Input: part model. Units: mm. Frame: model coordinates. A direction names the side the tool comes from. Coordinates: 2 decimals unless noted, no trailing zeros. Loops run counter-clockwise (first coordinate to the right, second up) from the corner with the lowest first, then second, coordinate; pieces in that order, holes last. Notation, with made-up numbers: (-35.5, 72.5) - (-8.5, 72.5) arc R13 ccw to (-8.5, 81.5) - close; hole circle Ø11 at (23, 53). An arc over 180 degrees is marked (long way). Write item = value, one per line. Start each with the question number.
from build123d import *

# Parameters (mm, degrees)
CHAMFER1_SIZE = 0.5


with BuildPart() as part:
    # Sketch1 → Revolve1 (revolve)
    with BuildSketch(Plane.XY):
        Polygon((3.925, 17.592522397), (6.15, 17.592522397), (6.15, 13.092522397), (9.15, 13.092522397), (9.15, 18.092522397), (11.15, 18.092522397), (11.15, 11.092522397), (9.662817283, 11.092522397), (3.925, 11.092522397), align=None)
    revolve(axis=Axis((0, 0, 0), (0, 1, 0)))

    # Chamfer1
    chamfer1_edges = [part.edges().sort_by_distance(p)[0] for p in [
        (-11.15, 18.092522397, 0),
        (-11.15, 11.092522397, 0),
    ]]
    chamfer(chamfer1_edges, length=CHAMFER1_SIZE)


solid = part.part
Item 1: Cut plane B-B on z = 0. Return loops of the section in (x, y) (3 decimals), plus the area to 3 significant figures.
Item 2: Pull-direction query (X, two-part tool) for faces 3 (the cylindrical face through (-2.893, 14.388, -2.653)), 4 (the flat face through (0, 11.093, 5)), 5 (the cylindrical face through (10.635, 14.551, -3.349)); classes: pulls with the +X half, pulls with the -X half, needs draft (parallel to the pull), parting line crosses it, or undercut.
Item 3: Cut plane A-A on x = 0. Return loops of the section in (y, z) (3 decimals).
Item 4: Cut plane C-C on y = 16.5. Return loops of the section in (x, z) (3 decimals), plus the area to 3 significant figures.
Item 5: Ray query, line 1 (X direction, y = 15.6, z = 0) (3 decimals); line 2 (Z direction, x = 2, y = 13.5). Return the intervals inside material, ascending.
Item 6: Access query for faces 1 (the flat face through (-5, 18.093, -8)), 2 (the cylindrical face through (4.919, 15.628, -7.715)). Directions: +Z, -Z, +X, -X, +Y, -Y. A direction counts if a zero-diameter tool reaches every point of the face in a straight line with its end or side. Return the directions, or none.
Item 7: Pin query (flat end, axial travel): pin 1 (2 mm diameter, centred on x = 2, y = 15.5, fed in from +Z); pin 2 (2 mm diameter, centred on y = 12.5, z = 3.5, fed in from +X); pin 3 (6 mm diameter, centred on x = 2.5, z = -4.5, fed in from +Y); pin 4 (7 mm diameter, centred on x = 0, z = 0, fed in from -Y). Return the tip coordinate at first contact, or that it passes through.
Recorded:
q1.outline = (-11.15, 11.593) - (-10.65, 11.093) - (-3.925, 11.093) - (-3.925, 17.593) - (-6.15, 17.593) - (-6.15, 13.093) - (-9.15, 13.093) - (-9.15, 18.093) - (-10.65, 18.093) - (-11.15, 17.593) - close; (3.925, 11.093) - (10.65, 11.093) - (11.15, 11.593) - (11.15, 17.593) - (10.65, 18.093) - (9.15, 18.093) - (9.15, 13.093) - (6.15, 13.093) - (6.15, 17.593) - (3.925, 17.593) - close
q1.area = 68.4 mm²
q2.face_3 = undercut
q2.face_4 = needs draft
q2.face_5 = parting line crosses it
q3.outline = (11.093, -10.65) - (11.593, -11.15) - (17.593, -11.15) - (18.093, -10.65) - (18.093, -9.15) - (13.093, -9.15) - (13.093, -6.15) - (17.593, -6.15) - (17.593, -3.925) - (11.093, -3.925) - close; (11.093, 3.925) - (17.593, 3.925) - (17.593, 6.15) - (13.093, 6.15) - (13.093, 9.15) - (18.093, 9.15) - (18.093, 10.65) - (17.593, 11.15) - (11.593, 11.15) - (11.093, 10.65) - close
q4.outline = circle Ø22.3 at (0, 0); circle Ø12.3 at (0, 0); hole circle Ø18.3 at (0, 0); hole circle Ø7.85 at (0, 0)
q4.area = 198 mm²
q5.line_1 = -11.15 to -9.15, -6.15 to -3.925, 3.925 to 6.15, 9.15 to 11.15
q5.line_2 = -10.97 to -8.93, -5.82 to -3.38, 3.38 to 5.82, 8.93 to 10.97
q6.face_1 = +Z, -Z, +X, -X, +Y
q6.face_2 = +Y
q7.pin_1 = 11.11
q7.pin_2 = 10.87
q7.pin_3 = 17.59
q7.pin_4 = through
